Read the model definition and answer for the solid it produces. Units are mm, in the model's axes. A direction names the side the tool comes from. Coordinates: 2 decimals unless noted, no trailing zeros. Loops run counter-clockwise (first coordinate to the right, second up) from the corner with the lowest first, then second, coordinate; pieces in that order, holes last. Notation, with made-up numbers: (45.25, 20) - (78.25, 20) arc R30 cw to (78.25, 56) - close; hole circle Ø7 at (70, 22). An arc over 180 degrees is marked (long way). One line per item, written item: value. Start each with the question number.
from build123d import *

# Parameters (mm, degrees)
SKETCH1_R           = 15
SKETCH1_R_2         = 6
BOSS_EXTRUDE1_DEPTH = 10
CUT_EXTRUDE1_DEPTH  = 24.452078799


with BuildPart() as part:
    # Sketch1 → Boss-Extrude1 (new body)
    with BuildSketch(Plane(origin=(0, 0, 0), x_dir=(1, 0, 0), z_dir=(0, 1, 0))):
        with Locations(Location((0, 0, 0), (0, 0, 270))):
            Circle(SKETCH1_R)
        with Locations(Location((0, 0, 0), (0, 0, 270))):
            Circle(SKETCH1_R_2, mode=Mode.SUBTRACT)
    extrude(amount=BOSS_EXTRUDE1_DEPTH)

    # Sketch2 → Cut-Extrude1 (cut, through all)
    with BuildSketch(Plane(origin=(0, 10, 0), x_dir=(1, 0, 0), z_dir=(0, 1, 0))):
        with BuildLine():
            Line((2, 5.656854249), (2, 7.656854249))
            Line((2, 7.656854249), (-2, 7.656854249))
            Line((-2, 7.656854249), (-2, 5.656854249))
            ThreePointArc((-2, 5.656854249), (0, 6), (2, 5.656854249))
        make_face()
    extrude(amount=-CUT_EXTRUDE1_DEPTH, mode=Mode.SUBTRACT)


solid = part.part
1) Straight lines are drawn through the part: L1, parallel to X at y = 6, z = 0; L2, parallel to Z at x = -5, y = 2.75; L3, parallel to Z at x = -1, y = 2. For each, find the intervals that lie inside material, in ascending order.
2) For faces 1 (the flat face through (0.2, 0, 6.5)), 2 (the flat face through (2, 5, -7)), determine the directions among +Z, -Z, +X, -X, +Y, -Y from which every point of the face is accessible in a straight line to the end or side of a thin tool.
3) Section D-D, the plane x = -8 is taken. Determine the outline of the cut face in (y, z).
4) Section C-C, the plane y = 4.25 is taken. Determine the outline of the cut face in (x, z), and give its area (3 significant figures).
5) Determine the mould class of faces 3 (the cylindrical face through (0.66, 4.93, -14.985)), 4 (the flat face through (0.2, 10, 6.5)), 5 (the cylindrical face through (0, 5, 6)) for opening direction Z: released by +Z, released by -Z, zero draft, split by the parting line, or undercut.
6) Section B-B, the plane x = 0 is taken. Determine the outline of the cut face in (y, z), and give its area (3 significant figures).
7) Flat-ended cylindrical pins translate along their axes: P1, Ø0.6, axis at y = 4, z = -7, coming from the -X side; P2, Ø7, axis at x = 0, z = 0, coming from the +Y side; P3, Ø3, axis at y = 7, z = -11.5, coming from the -X side; P4, Ø1, axis at y = 3.5, z = -6.5, coming from the +X side. Find the tip coordinate at first contact, or state that the pin passes through.
8) Section A-A, the plane z = 0 is taken. Determine the outline of the cut face in (x, y).
Answer below:
1. L1: -15 to -6, 6 to 15
1. L2: -14.14 to -3.32, 3.32 to 14.14
1. L3: -14.97 to -7.66, 5.92 to 14.97
2. face 1: +Z, -Z, +X, -X, -Y
2. face 2: +Y, -Y
3. outline: (0, -12.69) - (10, -12.69) - (10, 12.69) - (0, 12.69) - close
4. outline: circle Ø30 at (0, 0); hole (-2, -7.66) - (2, -7.66) - (2, -5.66) arc R6 ccw (long way) to (-2, -5.66) - close
4. area: 587 mm2
5. face 3: split by the parting line
5. face 4: zero draft
5. face 5: undercut
6. outline: (0, -15) - (10, -15) - (10, -7.66) - (0, -7.66) - close; (0, 6) - (10, 6) - (10, 15) - (0, 15) - close
6. area: 163 mm2
7. P1: x = -13.42
7. P2: through
7. P3: x = -11.18
7. P4: x = 13.75
8. outline: (-15, 0) - (-6, 0) - (-6, 10) - (-15, 10) - close; (6, 0) - (15, 0) - (15, 10) - (6, 10) - close
